```python
from build123d import *

# Parameters (mm, degrees)
EXTRUDE_1_DEPTH          = 5
EXTRUDE_1_DEPTH_BACK     = 5
SKETCH_1_R               = 1.5
CUT_EXTRUDE_1_DEPTH      = 3
CUT_EXTRUDE_1_DEPTH_BACK = 3
SKETCH_2_R               = 1.5
EXTRUDE_4_DEPTH          = 2.8
EXTRUDE_4_DEPTH_BACK     = 2.8
SKETCH_3_R               = 1.5
FILLET_1_R               = 10
FILLET_2_R               = 1
SCALE1_SCALE             = 1.5


with BuildPart() as part:
    # 草图1 → 凸台-拉伸1 (new, two sides: drawn at the far end of the back side and taken through both)
    with BuildSketch(Plane.XY.offset(-EXTRUDE_1_DEPTH_BACK)):
        with BuildLine():
            Line((255.314096956, 96.605744176), (199.091935004, 34.648006604))
            ThreePointArc((199.091935004, 34.648006604), (194.385791324, 34.210713053), (193.535103741, 38.859943595))
            Line((193.535103741, 38.859943595), (236.376857538, 107.153065983))
            Line((236.376857538, 107.153065983), (255.681175992, 119.525749162))
            ThreePointArc((255.681175992, 119.525749162), (259.048997407, 119.43741832), (260.211134207, 116.275225808))
            Line((260.211134207, 116.275225808), (255.314096956, 96.605744176))
        make_face()
        with Locations((196.5, 37)):
            Circle(SKETCH_1_R, mode=Mode.SUBTRACT)
        with Locations((202.248291042, 44.563540844)):
            Circle(SKETCH_1_R, mode=Mode.SUBTRACT)
        with Locations((257.3, 117)):
            Circle(SKETCH_1_R, mode=Mode.SUBTRACT)
        with Locations((240.118819851, 104.309174626)):
            Circle(SKETCH_1_R, mode=Mode.SUBTRACT)
    extrude(amount=EXTRUDE_1_DEPTH + EXTRUDE_1_DEPTH_BACK)

    # 草图2 → 切除-拉伸1 (cut, two sides: drawn at the far end of the back side and taken through both)
    with BuildSketch(Plane.XY.offset(-CUT_EXTRUDE_1_DEPTH_BACK)):
        with BuildLine():
            Line((255.681175992, 119.525749162), (242.27027225, 110.930322002))
            Line((242.27027225, 110.930322002), (258.937967915, 111.161415211))
            Line((258.937967915, 111.161415211), (260.211134207, 116.275225808))
            ThreePointArc((260.211134207, 116.275225808), (259.048997407, 119.43741832), (255.681175992, 119.525749162))
        make_face()
        with Locations((257.3, 117)):
            Circle(SKETCH_2_R, mode=Mode.SUBTRACT)
    extrude(amount=CUT_EXTRUDE_1_DEPTH + CUT_EXTRUDE_1_DEPTH_BACK, mode=Mode.SUBTRACT)

    # 草图3 → 凸台-拉伸4 (add, two sides: drawn at the far end of the back side and taken through both)
    with BuildSketch(Plane.XY.offset(-EXTRUDE_4_DEPTH_BACK)):
        with BuildLine():
            Line((244.560105761, 84.754670841), (247.522317194, 82.066678389))
            ThreePointArc((247.522317194, 82.066678389), (250.878196788, 81.678515203), (252.324623716, 84.731456021))
            Line((252.324623716, 84.731456021), (251.028481638, 91.882926341))
            Line((251.028481638, 91.882926341), (244.560105761, 84.754670841))
        make_face()
        with Locations((249.471111722, 84.214281678)):
            Circle(SKETCH_3_R, mode=Mode.SUBTRACT)
    extrude(amount=EXTRUDE_4_DEPTH + EXTRUDE_4_DEPTH_BACK)

    # 圆角1
    fillet_1_edges = [part.edges().sort_by_distance(p)[0] for p in [
        (236.376857538, 107.153065983, 0),
        (255.314096956, 96.605744176, 0),
    ]]
    fillet(fillet_1_edges, radius=FILLET_1_R)

    # 圆角2
    fillet_2_edges = [part.edges().sort_by_distance(p)[0] for p in [
        (258.937967915, 111.161415211, 0),
        (242.27027225, 110.930322002, 0),
    ]]
    fillet(fillet_2_edges, radius=FILLET_2_R)


with BuildPart() as part_1:
    # Scale1: scaled about (229.397572443, 79.796058166, 0)
    add(part.part.scale(SCALE1_SCALE).moved(Location((-114.698786222, -39.898029083, 0))))


solid = part_1.part
```
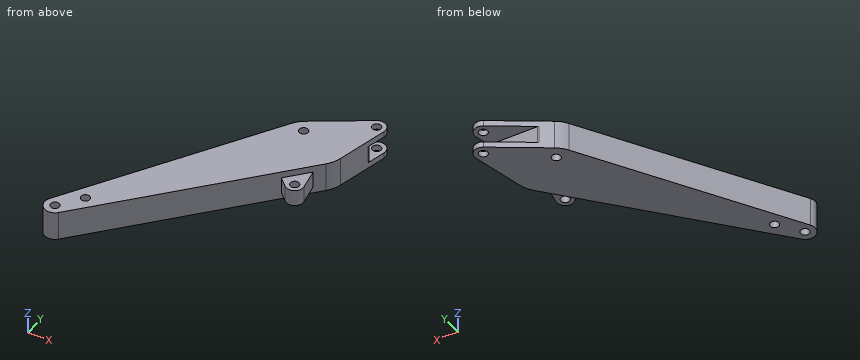
Check sheet for the modelled part. Datum: model origin and axes. Units: mm. Give positions to 0.01 mm unless a question says otherwise; leave off trailing zeros. Write each loop counter-clockwise with the first axis right and the second up, starting at its lowest first coordinate (ties: lowest second). Pieces come first, ordered by that corner, then holes.
Item 1: Cross-section at D-D (x = 208). Enter the section's corners in (y, z), and give its area (3 significant figures).
Item 2: Cross-section at C-C (x = 228.5). Enter the section's corners in (y, z), and give its area (3 significant figures).
Item 3: Cross-section at B-B (y = 96). Enter the section's corners in (x, z).
Item 4: Scan lines: L1, parallel to X at y = 82.5, z = -1.5; L2, parallel to Y at x = 180.5, z = 2.75; L3, parallel to Y at x = 219, z = -3.5. Record each from-to range of solid material in increasing order.
Item 5: Cross-section at A-A (z = 2). Enter the section's corners in (x, y).
Item 6: Gauge pin test, flat ends, axial feed: pin 1 (8 mm diameter, centred on y = 34.5, z = 3.5, fed in from -X); pin 2 (6 mm diameter, centred on x = 260.5, y = 91.5, fed in from -Z); pin 3 (8 mm diameter, centred on x = 197.5, z = 2, fed in from +Y); pin 4 (4 mm diameter, centred on x = 180.05, y = 15.6, fed in from -Z). Record the tip position at first contact, or that the pin passes through.
Report:
1. outline: (38.59, -7.5) - (70.03, -7.5) - (70.03, 7.5) - (38.59, 7.5) - close
1. area: 472 mm2
2. outline: (61.18, -7.5) - (102.71, -7.5) - (102.71, 7.5) - (61.18, 7.5) - close
2. area: 623 mm2
3. outline: (224.29, -7.5) - (260.1, -7.5) - (260.1, -4.2) - (262.19, -4.2) - (262.19, 4.2) - (260.1, 4.2) - (260.1, 7.5) - (224.29, 7.5) - close
4. L1: x = 215.82 to 247.85, 257.63 to 261.39
4. L2: y = 10.37 to 13.4, 17.81 to 26.2
4. L3: y = 50.71 to 87.57
5. outline: (175.6, 18.39) arc R5.25 ccw to (183.94, 12.07) - (252.14, 87.23) - (256.58, 83.2) arc R4.35 ccw to (263.79, 87.2) - (261.84, 97.93) - (265.74, 102.22) arc R15 ccw to (269.18, 108.67) - (273.24, 124.95) arc R1.5 ccw to (271.76, 126.82) - (249.13, 126.5) arc R1.5 ccw to (248.35, 126.27) - (242.69, 122.64) arc R15 ccw to (238.08, 117.99) - close; hole circle Ø4.5 at (180.05, 15.6); hole circle Ø4.5 at (188.67, 26.95); hole circle Ø4.5 at (245.48, 116.57); hole circle Ø4.5 at (259.51, 86.42)
6. pin 1: stops at x = 183.2
6. pin 2: stops at z = -4.2
6. pin 3: stops at y = 59.67
6. pin 4: passes through
